from build123d import *

# Parameters (mm, degrees)
SKETCH1_R           = 32.512
BOSS_EXTRUDE1_DEPTH = 1.905
SKETCH2_R           = 29.845
SKETCH2_R_2         = 27.305
BOSS_EXTRUDE2_DEPTH = 1.27
SKETCH3_R           = 9.525
BOSS_EXTRUDE3_DEPTH = 1.27
CUT_EXTRUDE1_REACH  = 48.136
CIRPATTERN1_COUNT   = 4
SKETCH5_R           = 2.54
SKETCH5_R_2         = 1.5875
BOSS_EXTRUDE4_DEPTH = 0.254
CUT_EXTRUDE2_REACH  = 48.451
SKETCH6_R           = 1.5875


with BuildPart() as part:
    # Sketch1 → Boss-Extrude1 (new, symmetric)
    with BuildSketch(Plane.XY):
        with Locations(Location((0, 0, 0), (0, 0, 180))):
            Circle(SKETCH1_R)
    extrude(amount=BOSS_EXTRUDE1_DEPTH, both=True)

    # Sketch2 → Boss-Extrude2 (add)
    with BuildSketch(Plane.XY.offset(1.905)):
        Circle(SKETCH2_R)
        Circle(SKETCH2_R_2, mode=Mode.SUBTRACT)
    boss_extrude2 = extrude(amount=BOSS_EXTRUDE2_DEPTH)

    # Sketch3 → Boss-Extrude3 (add)
    with BuildSketch(Plane.XY.offset(1.905)):
        Circle(SKETCH3_R)
    boss_extrude3 = extrude(amount=BOSS_EXTRUDE3_DEPTH)

    # Sketch4 → Cut-Extrude1 (cut, up to next)
    with BuildSketch(Plane.XY.offset(1.905), mode=Mode.PRIVATE) as cut_extrude1_sk1:
        with BuildLine():
            ThreePointArc((10.885714286, 19.366421534), (0, 21.8173208), (-10.885714286, 19.366421534))
            ThreePointArc((-10.885714286, 19.366421534), (-12.336421788, 15.022476336), (-7.9375, 13.748153285))
            Line((-7.9375, 13.748153285), (-7.931449378, 13.737673301))
            ThreePointArc((-7.931449378, 13.737673301), (0, 15.4673208), (7.931449378, 13.737673301))
            Line((7.931449378, 13.737673301), (7.9375, 13.748153285))
            ThreePointArc((7.9375, 13.748153285), (12.336421788, 15.022476336), (10.885714286, 19.366421534))
        make_face()
    cut_extrude1_tool1 = extrude(cut_extrude1_sk1.sketch, amount=-CUT_EXTRUDE1_REACH, mode=Mode.PRIVATE) & part.part
    cut_extrude1 = cut_extrude1_tool1.solids().sort_by_distance((0, 17.6348, 1.905))[0]
    add(cut_extrude1, mode=Mode.SUBTRACT)

    # CirPattern1: Cut-Extrude1 ×4 about axis
    cirpattern1_axis = Axis((0, 0, 0), (0, 0, 1))
    for i in range(1, CIRPATTERN1_COUNT):
        add(cut_extrude1.rotate(cirpattern1_axis, i * 360 / CIRPATTERN1_COUNT), mode=Mode.SUBTRACT)

    # Sketch5 → Boss-Extrude4 (add)
    with BuildSketch(Plane.XY.offset(3.175)):
        Circle(SKETCH5_R)
        Circle(SKETCH5_R_2, mode=Mode.SUBTRACT)
    boss_extrude4 = extrude(amount=BOSS_EXTRUDE4_DEPTH)

    # Mirror1: Boss-Extrude2, Boss-Extrude3, Boss-Extrude4 across plane
    add(boss_extrude2.mirror(Plane.XY))
    add(boss_extrude3.mirror(Plane.XY))
    add(boss_extrude4.mirror(Plane.XY))

    # Sketch6 → Cut-Extrude2 (cut, up to next)
    with BuildSketch(Plane.XY.offset(3.175), mode=Mode.PRIVATE) as cut_extrude2_sk1:
        Circle(SKETCH6_R)
    cut_extrude2_tool1 = extrude(cut_extrude2_sk1.sketch, amount=-CUT_EXTRUDE2_REACH, mode=Mode.PRIVATE) & part.part
    add(cut_extrude2_tool1.solids().sort_by_distance((0, 0, 3.175))[0], mode=Mode.SUBTRACT)


solid = part.part
For this review, take the finished solid that the model builds, in its own axes (mm). A direction names the side the tool comes from. Give positions to 0.01 mm unless a question says otherwise; leave off trailing zeros. Order: outer loops, then holes, each group sorted by start corner. A loop starts at its lowest first (then second) coordinate and runs counter-clockwise, first axis right, second up. Notation, with made-up numbers: (29, 26) - (34, 26) arc R21 ccw to (34, 42) - close; hole circle Ø7 at (31, 7.5). An arc over 180 degrees is marked (long way). Answer as a JSON object with one key per item and string values. Group by question number.
Item 1: Take a section at B-B on y = -14.5. Give the boundary of the cut face in (x, z) (3 decimals).
Item 2: Wall thickness on line 1 along Y through (x, z) = (0, 2.5) (1 decimal); line 2 along Y through (x, z) = (-1, -2.5); line 3 along Y through (x, z) = (-7.5, 0.75): over which ranges is each line inside the solid? List them lowest first.
Item 3: Draft analysis for pull direction Y (two halves, no side actions). For faces 4 (the cylindrical face through (14.959, -12.302, 0.027)), 5 (the flat face through (0, -2, 3.429)), 6 (the cylindrical face through (28.47, 8.96, -2.53)), state which applies: pulls with the +Y half, pulls with the -Y half, needs draft (parallel to the pull), parting line crosses it, or undercut.
Item 4: Take a section at A-A on z = -0.75. Give the number of separate pieces and of enclosed holes in the cut face, and give its area (3 significant figures).
Item 5: Clearance check with flat-ended pins moving along their axes: pin 1 Ø1.5 at (y, z) = (1, -1.5) entering from -X; pin 2 Ø4 at (y, z) = (6, 2.5) entering from -X; pin 3 Ø5.5 at (x, y) = (3.5, 2) entering from +Z; pin 4 Ø12 at (x, y) = (12.5, -14) entering from -Z (3 decimals). State where each tip first meets the part, or that it passes through.
Item 6: Machinability: for faces 1 (the cylindrical face through (0.157, 21.817, 0.027)), 2 (the flat face through (2, -2, 3.175)), 3 (the flat face through (-29, 9, -1.905)), which of the approach directions +Z, -Z, +X, -X, +Y, -Y give a long, thin tool a straight path to every point of the face, cutting with its end or side? Answer none if there is none.
Reported:
{
 "1": {"outline": "(-29.099, -1.905) - (-26.086, -1.905) - (-26.086, -3.175) - (-23.137, -3.175) - (-23.137, -1.905) - (-11.993, -1.905) - (-11.993, 1.905) - (-23.137, 1.905) - (-23.137, 3.175) - (-26.086, 3.175) - (-26.086, 1.905) - (-29.099, 1.905) - close; (-5.993, -1.905) - (5.993, -1.905) - (5.993, 1.905) - (-5.993, 1.905) - close; (11.993, -1.905) - (23.137, -1.905) - (23.137, -3.175) - (26.086, -3.175) - (26.086, -1.905) - (29.099, -1.905) - (29.099, 1.905) - (26.086, 1.905) - (26.086, 3.175) - (23.137, 3.175) - (23.137, 1.905) - (11.993, 1.905) - close"},
 "2": {"line 1": "-29.8 to -27.3, -9.5 to -1.6, 1.6 to 9.5, 27.3 to 29.8", "line 2": "-29.83 to -27.29, -9.47 to -1.23, 1.23 to 9.47, 27.29 to 29.83", "line 3": "-31.64 to -20.68, -13.93 to 13.93, 20.68 to 31.64"},
 "3": {"face 4": "undercut", "face 5": "needs draft", "face 6": "parting line crosses it"},
 "4": {"separate pieces": "1", "enclosed holes": "5", "area": "2,690 mm^2"},
 "5": {"pin 1": "x = -32.51", "pin 2": "x = -32.25", "pin 3": "z = 3.43", "pin 4": "z = -1.905"},
 "6": {"face 1": "+Z, -Z", "face 2": "+Z", "face 3": "-Z"}
}
